from build123d import *

# Parameters (mm, degrees)
SKETCH1_R           = 14
BOSS_EXTRUDE1_DEPTH = 2
SKETCH2_R           = 14
SKETCH2_R_2         = 4
BOSS_EXTRUDE2_DEPTH = 7.5
SKETCH3_R           = 7.5
CUT_EXTRUDE1_DEPTH  = 2
SKETCH5_R           = 1.25
CUT_EXTRUDE2_DEPTH  = 22.960191256
SKETCH7_R           = 1.75
CUT_EXTRUDE3_DEPTH  = 15
SKETCH9_R           = 1.75
CUT_EXTRUDE4_DEPTH  = 15
SKETCH10_R          = 2.25
CUT_EXTRUDE5_DEPTH  = 2
SKETCH11_R          = 2.75
CUT_EXTRUDE6_DEPTH  = 2
SKETCH12_R          = 2.75
CUT_EXTRUDE7_DEPTH  = 2


with BuildPart() as part:
    # Sketch1 → Boss-Extrude1 (new body)
    with BuildSketch(Plane.XY):
        Circle(SKETCH1_R)
    extrude(amount=BOSS_EXTRUDE1_DEPTH)

    # Sketch2 → Boss-Extrude2 (add)
    with BuildSketch(Plane.XY.offset(2)):
        Circle(SKETCH2_R)
        Circle(SKETCH2_R_2, mode=Mode.SUBTRACT)
    extrude(amount=BOSS_EXTRUDE2_DEPTH)

    # Sketch3 → Cut-Extrude1 (cut)
    with BuildSketch(Plane(origin=(0, 0, 0), x_dir=(-1, 0, 0), z_dir=(0, 0, -1))):
        Circle(SKETCH3_R)
    extrude(amount=-CUT_EXTRUDE1_DEPTH, mode=Mode.SUBTRACT)

    # Sketch5 → Cut-Extrude2 (cut, through all)
    with BuildSketch(Plane.XY.offset(9.5)):
        with Locations((0, 10.75)):
            Circle(SKETCH5_R)
        with Locations((10.75, 0)):
            Circle(SKETCH5_R)
        with Locations((0, -10.75)):
            Circle(SKETCH5_R)
        with Locations((-10.75, 0)):
            Circle(SKETCH5_R)
    extrude(amount=-CUT_EXTRUDE2_DEPTH, mode=Mode.SUBTRACT)

    # Sketch7 → Cut-Extrude3 (cut)
    with BuildSketch(Plane(origin=(9.899494937, 9.899494937, 0), x_dir=(0.7071067811865489, -0.7071067811865461, 0), z_dir=(0.7071067811865461, 0.7071067811865489, 0))):
        with Locations(Location((0, -4.75, 0), (0, 0, 180))):
            Circle(SKETCH7_R)
    extrude(amount=-CUT_EXTRUDE3_DEPTH, mode=Mode.SUBTRACT)

    # Sketch9 → Cut-Extrude4 (cut)
    with BuildSketch(Plane(origin=(-9.899494937, 9.899494937, 0), x_dir=(0, 0, 1), z_dir=(-0.7071067811865489, 0.7071067811865462, 0))):
        with Locations(Location((5, 0, 0), (0, 0, 270))):
            Circle(SKETCH9_R)
    extrude(amount=-CUT_EXTRUDE4_DEPTH, mode=Mode.SUBTRACT)

    # Sketch10 → Cut-Extrude5 (cut)
    with BuildSketch(Plane.XY.offset(9.5)):
        with Locations((0, 10.75)):
            Circle(SKETCH10_R)
        with Locations((10.75, 0)):
            Circle(SKETCH10_R)
        with Locations((0, -10.75)):
            Circle(SKETCH10_R)
        with Locations((-10.75, 0)):
            Circle(SKETCH10_R)
    extrude(amount=-CUT_EXTRUDE5_DEPTH, mode=Mode.SUBTRACT)

    # Sketch11 → Cut-Extrude6 (cut)
    with BuildSketch(Plane(origin=(9.899494937, 9.899494937, 0), x_dir=(0.7071067811865489, -0.7071067811865461, 0), z_dir=(0.7071067811865461, 0.7071067811865489, 0))):
        with Locations(Location((0, -4.75, 0), (0, 0, 180))):
            Circle(SKETCH11_R)
    extrude(amount=-CUT_EXTRUDE6_DEPTH, mode=Mode.SUBTRACT)

    # Sketch12 → Cut-Extrude7 (cut)
    with BuildSketch(Plane(origin=(-9.899494937, 9.899494937, 0), x_dir=(0, 0, 1), z_dir=(-0.7071067811865489, 0.7071067811865462, 0))):
        with Locations(Location((5, 0, 0), (0, 0, 270))):
            Circle(SKETCH12_R)
    extrude(amount=-CUT_EXTRUDE7_DEPTH, mode=Mode.SUBTRACT)


solid = part.part
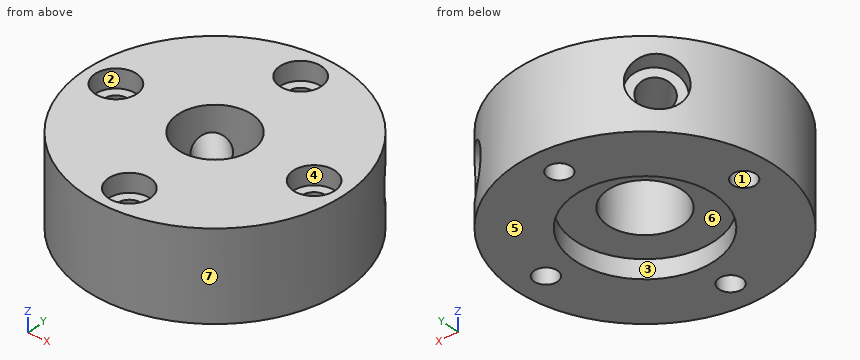
The listing builds one solid part. Answer for the finished solid, in the listing's coordinates (mm). Face numbers are marked on the shaded views. A direction names the side the tool comes from. Coordinates: 2 decimals unless noted, no trailing zeros. Loops run counter-clockwise (first coordinate to the right, second up) from the corner with the lowest first, then second, coordinate; pieces in that order, holes last. Notation, with made-up numbers: (37.5, 85.25) -> (58.5, 85.25) arc R20 cw to (58.5, 100.25) -> close; hole circle Ø7 at (60, -12). An arc over 180 degrees is marked (long way). Answer in a Markdown table with one row per item. Add a question column.
1. Determine the mould class of the marked faces 4, 5, 6 and 7 for opening direction Y: +Y half, -Y half, draft (parallel to the pull), parting line (faces both ways), or undercut.
2. The part is cut by section D-D, the plane y = -11.5. Write down the section's boundary in (x, z).
3. Consider line 1 (Y direction, x = 0, z = 4.75); line 2 (Z direction, x = -8.75, y = 9); line 3 (X direction, y = 1, z = 3). Determine where each line is inside the solid, lowest interval first. Write a range as [from, to].
4. Flat-ended cylindrical pins translate along their axes: P1, Ø6.5, axis at x = 0, y = 0, coming from the -Z side; P2, Ø4, axis at y = 4.5, z = 6.5, coming from the +X side (3 decimals); P3, Ø9, axis at x = 0, y = 0, coming from the -Z side; P4, Ø3, axis at x = -10.75, y = 0, coming from the +Z side. Find the tip coordinate at first contact, or state that the pin passes through.
5. The part is cut by section C-C, the plane z = 5.75. Write down the section's boundary in (x, y), then the cut area to 3 significant figures.
6. For the marked faces 1, 2 and 3, determine the directions among +Z, -Z, +X, -X, +Y, -Y from which every point of the face is accessible in a straight line to the end or side of a thin tool.
7. The part is cut by section A-A, the plane x = 0. Write down the section's boundary in (y, z).
Answer below:
| question | item | result |
|---|---|---|
| 1 | face 4 | undercut |
| 1 | face 5 | draft |
| 1 | face 6 | undercut |
| 1 | face 7 | parting line |
| 2 | outline | (-7.98, 0) -> (-1, 0) -> (-1, 7.5) -> (-2.12, 7.5) -> (-2.12, 9.5) -> (-7.98, 9.5) -> close; (1, 0) -> (7.98, 0) -> (7.98, 9.5) -> (2.12, 9.5) -> (2.12, 7.5) -> (1, 7.5) -> close |
| 3 | line 1 | [-14, -12], [-9.5, -4], [4, 9.5], [12, 14] |
| 3 | line 2 | [0, 2.26], [7.74, 9.5] |
| 3 | line 3 | [-13.96, -11.5], [-10, -3.87], [3.87, 10], [11.5, 13.96] |
| 4 | P1 | through |
| 4 | P2 | x = 13.775 |
| 4 | P3 | z = 2 |
| 4 | P4 | z = 7.5 |
| 5 | outline | (-11.59, 7.85) arc R14 ccw (long way) to (11.54, 7.92) -> (10.3, 6.67) -> (9.5, 7.47) -> (3.66, 1.62) arc R4 cw (long way) to (-3.72, 1.48) -> (-9.6, 7.37) -> (-10.36, 6.61) -> close; (-7.85, 11.59) -> (-6.61, 10.36) -> (-7.37, 9.6) -> (-1.48, 3.72) arc R4 cw to (1.62, 3.66) -> (7.47, 9.5) -> (6.67, 10.3) -> (7.92, 11.54) arc R14 ccw to start; hole circle Ø2.5 at (-10.75, 0); hole circle Ø2.5 at (0, -10.75); hole circle Ø2.5 at (0, 10.75); hole circle Ø2.5 at (10.75, 0) |
| 5 | area | 477 mm2 |
| 6 | face 1 | +Z, -Z |
| 6 | face 2 | +Z |
| 6 | face 3 | -Z |
| 7 | outline | (-14, 0) -> (-12, 0) -> (-12, 7.5) -> (-13, 7.5) -> (-13, 9.5) -> (-14, 9.5) -> close; (-9.5, 0) -> (-7.5, 0) -> (-7.5, 2) -> (-4, 2) -> (-4, 9.5) -> (-8.5, 9.5) -> (-8.5, 7.5) -> (-9.5, 7.5) -> close; (4, 2) -> (7.5, 2) -> (7.5, 0) -> (9.5, 0) -> (9.5, 7.5) -> (8.5, 7.5) -> (8.5, 9.5) -> (4, 9.5) -> close; (12, 0) -> (14, 0) -> (14, 9.5) -> (13, 9.5) -> (13, 7.5) -> (12, 7.5) -> close |
